from build123d import *

# Parameters (mm, degrees)
CYLINDER004_R                       = 1.9
CYLINDER004_DEPTH                   = 10
BOX011_W                            = 8.2
BOX011_H                            = 24
BOX011_DEPTH                        = 5
BOX012_W                            = 15
BOX012_H                            = 21
BOX012_DEPTH                        = 17
CHAMFER013_SIZE2                    = 16.5
CHAMFER013_SIZE                     = 9
BOX010_W                            = 12.5
BOX010_H                            = 21.5
BOX010_DEPTH                        = 10
CHAMFER009_SIZE2                    = 2.5
CHAMFER009_SIZE                     = 4
BOX008_W                            = 12.5
BOX008_H                            = 20
BOX008_DEPTH                        = 9
CHAMFER010_SIZE                     = 4
CHAMFER012_SIZE2                    = 8.5
CHAMFER012_SIZE                     = 16.5
BOX013_W                            = 3
BOX013_H                            = 24.5
BOX013_DEPTH                        = 5
CHAMFER023004_SIZE2                 = 24
CHAMFER023004_SIZE                  = 4
BOX009_W                            = 10
BOX009_H                            = 23.5
BOX009_DEPTH                        = 5
CHAMFER023003_SIZE                  = 1
CYLINDER002_R                       = 1.65
CYLINDER002_DEPTH                   = 10
CYLINDER003_R                       = 1.65
CYLINDER003_DEPTH                   = 10
BOX007_W                            = 4
BOX007_H                            = 16
BOX007_DEPTH                        = 8
CHAMFER011_SIZE                     = 1.5
CHAMFER023006002_SIZE               = 0.4
CHAMFER023006003_SIZE               = 0.2
CHAMFER023006003001_PLACEMENT_ANGLE = 90


with BuildPart() as cylinder004:
    # Cylinder004 → Cylinder004 (new body)
    with BuildSketch(Plane(origin=(-3.5, -12.25, 10), x_dir=(1, 0, 0), z_dir=(0, 0, 1))):
        Circle(CYLINDER004_R)
    extrude(amount=CYLINDER004_DEPTH)


with BuildPart() as cube011:
    # Box011 → Box011 (new body)
    with BuildSketch(Plane(origin=(-7.6, -28.5, 16), x_dir=(1, 0, 0), z_dir=(0, 0, 1))):
        with Locations((4.1, 12)):
            Rectangle(BOX011_W, BOX011_H)
    extrude(amount=BOX011_DEPTH)


with BuildPart() as chamfer013:
    # Box012 → Box012 (new body)
    with BuildSketch(Plane(origin=(-10.8, -4.5, 8), x_dir=(1, 0, 0), z_dir=(0, 0, 1))):
        with Locations((7.5, 10.5)):
            Rectangle(BOX012_W, BOX012_H)
    extrude(amount=BOX012_DEPTH)

    # Chamfer013
    chamfer013_edges = [chamfer013.edges().sort_by_distance(p)[0] for p in [
        (-3.3, -4.5, 8),
    ]]
    chamfer013_side = chamfer013.faces().sort_by_distance((-3.3, -4.5, 16.5))[0]
    chamfer(chamfer013_edges, length=CHAMFER013_SIZE, length2=CHAMFER013_SIZE2, reference=chamfer013_side)


with BuildPart() as chamfer009:
    # Box010 → Box010 (new body)
    with BuildSketch(Plane(origin=(1.5, -9.5, 8), x_dir=(1, 0, 0), z_dir=(0, 0, 1))):
        with Locations((6.25, 10.75)):
            Rectangle(BOX010_W, BOX010_H)
    extrude(amount=BOX010_DEPTH)

    # Chamfer009
    chamfer009_edges = [chamfer009.edges().sort_by_distance(p)[0] for p in [
        (1.5, 1.25, 8),
    ]]
    chamfer009_side = chamfer009.faces().sort_by_distance((1.5, 1.25, 13))[0]
    chamfer(chamfer009_edges, length=CHAMFER009_SIZE, length2=CHAMFER009_SIZE2, reference=chamfer009_side)


with BuildPart() as cut003001004:
    # Box008 → Box008 (new body)
    with BuildSketch(Plane(origin=(-8.5, -8, 8), x_dir=(1, 0, 0), z_dir=(0, 0, 1))):
        with Locations((6.25, 10)):
            Rectangle(BOX008_W, BOX008_H)
    extrude(amount=BOX008_DEPTH)

    # Chamfer010
    chamfer010_edges = [cut003001004.edges().sort_by_distance(p)[0] for p in [
        (-2.25, -8, 8),
    ]]
    chamfer(chamfer010_edges, length=CHAMFER010_SIZE)

    # Cut003001002: cut Chamfer009
    add(chamfer009.part, mode=Mode.SUBTRACT)

    # Chamfer012
    chamfer012_edges = [cut003001004.edges().sort_by_distance(p)[0] for p in [
        (-8.5, 12, 12.5),
    ]]
    chamfer012_side = cut003001004.faces().sort_by_distance((-8.5, 2.403101, 12.647287))[0]
    chamfer(chamfer012_edges, length=CHAMFER012_SIZE, length2=CHAMFER012_SIZE2, reference=chamfer012_side)

    # Cut003001004: cut Chamfer013
    add(chamfer013.part, mode=Mode.SUBTRACT)


with BuildPart() as chamfer023004:
    # Box013 → Box013 (new body)
    with BuildSketch(Plane(origin=(-1.5, -3.5, 13), x_dir=(1, 0, 0), z_dir=(0, 0, -1))):
        with Locations((1.5, 12.25)):
            Rectangle(BOX013_W, BOX013_H)
    extrude(amount=BOX013_DEPTH)

    # Chamfer023004
    chamfer023004_edges = [chamfer023004.edges().sort_by_distance(p)[0] for p in [
        (0, -28, 8),
    ]]
    chamfer023004_side = chamfer023004.faces().sort_by_distance((0, -28, 10.5))[0]
    chamfer(chamfer023004_edges, length=CHAMFER023004_SIZE, length2=CHAMFER023004_SIZE2, reference=chamfer023004_side)


with BuildPart() as chamfer023003:
    # Box009 → Box009 (new body)
    with BuildSketch(Plane(origin=(-8.5, -28, 12), x_dir=(1, 0, 0), z_dir=(0, 0, 1))):
        with Locations((5, 11.75)):
            Rectangle(BOX009_W, BOX009_H)
    extrude(amount=BOX009_DEPTH)

    # Chamfer023003
    chamfer023003_edges = [chamfer023003.edges().sort_by_distance(p)[0] for p in [
        (-8.5, -16.25, 12),
        (1.5, -16.25, 12),
    ]]
    chamfer(chamfer023003_edges, length=CHAMFER023003_SIZE)


with BuildPart() as cylinder002:
    # Cylinder002 → Cylinder002 (new body)
    with BuildSketch(Plane(origin=(0, 0, 4), x_dir=(0, 0, -1), z_dir=(1, 0, 0))):
        Circle(CYLINDER002_R)
    extrude(amount=CYLINDER002_DEPTH)


with BuildPart() as fusion001003:
    # Cylinder003 → Cylinder003 (new body)
    with BuildSketch(Plane(origin=(0, 8, 4), x_dir=(0, 0, -1), z_dir=(1, 0, 0))):
        Circle(CYLINDER003_R)
    extrude(amount=CYLINDER003_DEPTH)

    # Fusion001003: union Cylinder002
    add(cylinder002.part)


with BuildPart() as chamfer023006003001:
    # Box007 → Box007 (new body)
    with BuildSketch(Plane(origin=(0, -4, 0), x_dir=(1, 0, 0), z_dir=(0, 0, 1))):
        with Locations((2, 8)):
            Rectangle(BOX007_W, BOX007_H)
    extrude(amount=BOX007_DEPTH)

    # Chamfer011
    chamfer011_edges = [chamfer023006003001.edges().sort_by_distance(p)[0] for p in [
        (2, -4, 0),
        (2, 12, 0),
    ]]
    chamfer(chamfer011_edges, length=CHAMFER011_SIZE)

    # Cut003001003: cut Fusion001003
    add(fusion001003.part, mode=Mode.SUBTRACT)

    # Fusion001004: union Cut003001004, Chamfer023004, Chamfer023003
    add(cut003001004.part)
    add(chamfer023004.part)
    add(chamfer023003.part)

    # Cut003001015: cut Cube011
    add(cube011.part, mode=Mode.SUBTRACT)

    # Cut003001016: cut Cylinder004
    add(cylinder004.part, mode=Mode.SUBTRACT)

    # Chamfer023006002
    chamfer023006002_edges = [chamfer023006003001.edges().sort_by_distance(p)[0] for p in [
        (-5.4, -12.25, 16),
    ]]
    chamfer(chamfer023006002_edges, length=CHAMFER023006002_SIZE)

    # Chamfer023006003
    chamfer023006003_edges = [chamfer023006003001.edges().sort_by_distance(p)[0] for p in [
        (0, 8, 5.65),
        (0, 0, 5.65),
        (4, 8, 5.65),
        (4, 0, 5.65),
    ]]
    chamfer(chamfer023006003_edges, length=CHAMFER023006003_SIZE)


with BuildPart() as chamfer023006003001_1:
    # Chamfer023006003001 placement: moved
    add(chamfer023006003001.part.rotate(Axis((0, 0, 0), (-1, 0, 0)), CHAMFER023006003001_PLACEMENT_ANGLE))


solid = chamfer023006003001_1.part
CAD build for the part. Positions are in the model's coordinates, mm. A direction names the side the tool comes from. Round coordinates to 2 decimals unless told otherwise and drop trailing zeros. Loops run counter-clockwise (first coordinate to the right, second up) from the corner with the lowest first, then second, coordinate; pieces in that order, holes last.
(1) Drop flat-ended pins along their axis: pin 1 (5 mm diameter, centred on x = -6, z = 20.5, fed in from -Y); pin 2 (2 mm diameter, centred on x = -0.5, z = -0.5, fed in from +Y); pin 3 (4 mm diameter, centred on x = -3, z = 15, fed in from +Y). Give the stop position or say it passes through.
(2) Cut at C-C (x = -3.5). Give the cut face in (y, z).
(3) Which spindle directions (+Z, -Z, +X, -X, +Y, -Y) get a long thin tool onto all of the face, cutting with end or side? Do faces 1 (the flat face through (-5, 12, 18)), 2 (the cylindrical face through (1.97, 5.65, -0.07)). Say none if no direction does.
(4) Cut at A-A (y = 4). Give the cut face in (x, z).
(5) Wall check: line 1 along Z through (x, y) = (1.3, 4); line 2 along Y through (x, z) = (-1.75, 26.5); line 3 along X through (y, z) = (11.25, 14.5). Give the ranges that are in metal, low to high.
(6) Cut at B-B (z = 12.25). Give the cut face in (x, y) (3 decimals).
(7) Two-plate mould, pull along X, no slides. Class faces 3 (the flat face through (2, 5, 4)), 4 (the flat face through (-3.6, 16.5, 4.5)), 5 (the flat face through (-7.6, 16.5, 16.4)), 6 (the flat face through (-8.5, 15, 16)): +X half, -X half, draft (parallel to the pull), parting line (faces both ways), or undercut.
(8) Cut at D-D (y = 9.5). Give the cut face in (x, z), plus the area to 3 significant figures.
Findings below:
1. pin 1: stops at y = 12
1. pin 2: stops at y = 14.82
1. pin 3: stops at y = 16
2. outline: (8, -5.21) - (11.71, -5.21) - (17, 4.5) - (16, 4.5) - (16, 9.95) - (15.6, 10.35) - (12, 10.35) - (12, 8) - (8, 4) - close; (12, 14.15) - (15.6, 14.15) - (16, 14.55) - (16, 28) - (12, 28) - close
3. face 1: +Z, -X, -Y
3. face 2: +X, -X
4. outline: (0, -12) - (4, -12) - (4, -9.85) - (3.8, -9.65) - (0.2, -9.65) - (0, -9.85) - close; (0, -6.15) - (0.2, -6.35) - (3.8, -6.35) - (4, -6.15) - (4, -1.85) - (3.8, -1.65) - (0.2, -1.65) - (0, -1.85) - close; (0, 1.85) - (0.2, 1.65) - (3.8, 1.65) - (4, 1.85) - (4, 4) - (0, 4) - close
5. line 1: z = -12 to -9.65, -6.35 to -1.65, 1.65 to 4
5. line 2: y = 12 to 16
5. line 3: x = -1.5 to 1.5
6. outline: (-8.5, 13) - (-7.5, 12) - (-5.4, 12) - (-5.4, 15.6) - (-5.8, 16) - (-7.6, 16) - (-7.6, 17) - (-8.5, 17) - close; (-1.6, 12) - (-1.5, 12) - (-1.5, 9.375) - (1.5, 9.375) - (1.5, 17) - (0.6, 17) - (0.6, 16) - (-1.2, 16) - (-1.6, 15.6) - close
7. face 3: draft
7. face 4: undercut
7. face 5: undercut
7. face 6: -X half
8. outline: (-8.5, 4.5) - (-1.42, -9.25) - (3.06, -9.25) - (3.06, 5.5) - (1.5, 5.5) - (1.5, 13) - (-1.5, 13) - (-1.5, 5.5) - (-8.5, 5.5) - close
8. area: 144 mm2
